Verification items for the finished model (mm, model axes). A direction names the side the tool comes from. Coordinates: 2 decimals unless noted, no trailing zeros. Order: outer loops, then holes, each group sorted by start corner. A loop starts at its lowest first (then second) coordinate and runs counter-clockwise, first axis right, second up. Notation, with made-up numbers: M 20.25,36 L 42.25,36 A30 cw 42.25,58 Z; hole C 68.25,-26.75 d6. An arc over 180 degrees is marked long. Write item = value, one per line.
```python
from build123d import *

# Parameters (mm, degrees)
BOSS_EXTRUDE1_DEPTH = 15
CUT_EXTRUDE1_DEPTH  = 39.160843806
CUT_EXTRUDE2_DEPTH  = 38.762415177
CUT_EXTRUDE4_DEPTH  = 0.2
FILLET1_R           = 3


with BuildPart() as part:
    # Sketch2 → Boss-Extrude1 (new body)
    with BuildSketch(Plane.XY):
        Polygon((0, 0), (29.5, 0), (29.5, 5), (25, 5), (25, 24), (20, 24), (20, 5), (0, 5), align=None)
    extrude(amount=BOSS_EXTRUDE1_DEPTH)

    # Sketch3 → Cut-Extrude1 (cut, through all)
    with BuildSketch(Plane(origin=(0, 5, 0), x_dir=(1, 0, 0), z_dir=(0, 1, 0))):
        Polygon((10.25, -5.91228676), (7.5, -4.324573519), (4.75, -5.91228676), (4.75, -9.08771324), (7.5, -10.675426481), (10.25, -9.08771324), align=None)
        Polygon((44.25, -9.08771324), (44.25, -5.91228676), (47, -4.324573519), (49.75, -5.91228676), (49.75, -9.08771324), (47, -10.675426481), align=None)
    extrude(amount=-CUT_EXTRUDE1_DEPTH, mode=Mode.SUBTRACT)

    # Sketch4 → Cut-Extrude2 (cut, through all)
    with BuildSketch(Plane(origin=(25, 0, 0), x_dir=(0, 0, -1), z_dir=(1, 0, 0))):
        Polygon((-5.91228676, 11.9), (-4.324573519, 14.65), (-5.91228676, 17.4), (-9.08771324, 17.4), (-10.675426481, 14.65), (-9.08771324, 11.9), align=None)
    extrude(amount=-CUT_EXTRUDE2_DEPTH, mode=Mode.SUBTRACT)

    # Sketch5 → Cut-Extrude4 (cut)
    with BuildSketch(Plane(origin=(0, 0, 0), x_dir=(-1, 0, 0), z_dir=(0, 0, -1))):
        Polygon((-24.7, 4.7), (-24.7, 23.7), (-24.7, 24), (-25, 24), (-25, 5), (-29.5, 5), (-29.5, 4.7), align=None)
    extrude(amount=-CUT_EXTRUDE4_DEPTH, mode=Mode.SUBTRACT)

    # Fillet1
    fillet1_edges = [part.edges().sort_by_distance(p)[0] for p in [
        (20, 5, 7.5),
    ]]
    fillet(fillet1_edges, radius=FILLET1_R)


solid = part.part
```
Item 1: Scan lines: L1, parallel to Y at x = 24.75, z = 8; L2, parallel to X at y = 2, z = 6.5; L3, parallel to Z at x = 6.75, y = 2. Record each from-to range of solid material in increasing order. Write a range as from..to.
Report:
L1 = 0..11.9, 17.4..24
L2 = 0..4.75, 10.25..29.5
L3 = 0..4.76, 10.24..15
Item 2: Tool access check on faces 5 (the flat face through (4.75, 3, 7)), 6 (the flat face through (23, 24, 7)), 7 (the flat face through (22.54, 16.01, 5.11)). Record the directions out of +Z, -Z, +X, -X, +Y, -Y that give a thin tool (end or side, any length) a straight path to the whole face; none if there is none.
Report:
face_5 = +Y, -Y
face_6 = +Z, -Z, +X, -X, +Y
face_7 = +X, -X
Item 3: Sectioned sample at B-B, the plane y = 3. Enter the section's corners in (x, z), then the cut area to 3 significant figures.
Report:
outline = M 0,0 L 29.5,0 L 29.5,15 L 0,15 Z; hole M 4.75,5.91 L 7.5,4.32 L 10.25,5.91 L 10.25,9.09 L 7.5,10.68 L 4.75,9.09 Z
area = 416 mm^2
Item 4: Sectioned sample at D-D, the plane y = 13.25. Enter the section's corners in (x, z), then the cut area to 3 significant figures.
Report:
outline = M 20,0 L 24.7,0 L 24.7,0.2 L 25,0.2 L 25,5.13 L 20,5.13 Z; M 20,9.87 L 25,9.87 L 25,15 L 20,15 Z
area = 51.3 mm^2
Item 5: Sectioned sample at C-C, the plane z = 11.5. Enter the section's corners in (x, y), then the cut area to 3 significant figures.
Report:
outline = M 0,0 L 29.5,0 L 29.5,5 L 25,5 L 25,24 L 20,24 L 20,8 A3 cw 17,5 L 0,5 Z
area = 244 mm^2
Item 6: Gauge pin test, flat ends, axial feed: pin 1 (4.5 mm diameter, centred on y = 15, z = 10.5, fed in from +X); pin 2 (1 mm diameter, centred on y = 9, z = 2, fed in from -X); pin 3 (1.3 mm diameter, centred on x = 27.5, z = 9.5, fed in from +Y). Record the tip position at first contact, or that the pin passes through.
Report:
pin_1 = 25
pin_2 = 20
pin_3 = 5
Item 7: Release check for a two-part mould opening along X. For faces 1 (the flat face through (29.5, 2, 7)), 2 (the flat face through (20, 18, 7)), 3 (the flat face through (27, 5, 7)), 4 (the flat face through (8.86, 2.54, 9.89)) record: pulls with the +X half, pulls with the -X half, needs draft (parallel to the pull), parting line crosses it, or undercut.
Report:
face_1 = pulls with the +X half
face_2 = pulls with the -X half
face_3 = needs draft
face_4 = undercut
Item 8: Sectioned sample at A-A, the plane x = 22.75. Enter the section's corners in (y, z).
Report:
outline = M 0,0 L 24,0 L 24,15 L 0,15 Z; hole M 11.9,5.91 L 14.65,4.32 L 17.4,5.91 L 17.4,9.09 L 14.65,10.68 L 11.9,9.09 Z
